Part print with two shaded views. Sizes in mm from the minimum x, y, z corner. Round coordinates to 2 decimals unless told otherwise and drop trailing zeros. Order: outer loops, then holes, each group sorted by start corner. A loop starts at its lowest first (then second) coordinate and runs counter-clockwise, first axis right, second up. Notation, with made-up numbers: M 61,5.5 L 110,5.5 A25 cw 110,29.5 Z; hole C -37,12 d6. An arc over 180 degrees is marked long. Answer as a JSON object with one key per item and string values.
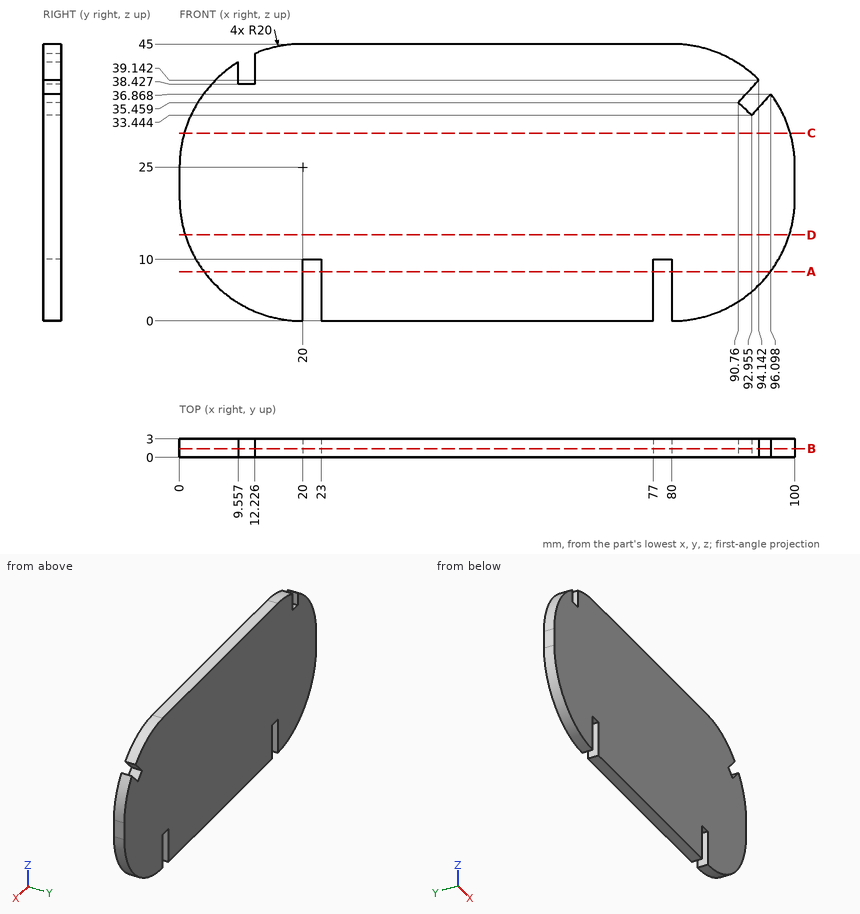
Item 1: Saw through at A-A on z = 8. List the corners of the cut face in (x, y).
Worked answers:
{"outline": "M 4,0 L 20,0 L 20,3 L 4,3 Z; M 23,0 L 77,0 L 77,3 L 23,3 Z; M 80,0 L 96,0 L 96,3 L 80,3 Z"}
Item 2: Drop flat-ended pins along their axis: pin 1 Ø1.5 at (y, z) = (1, 41) entering from -X; pin 2 Ø1.5 at (y, z) = (2, 7) entering from +X; pin 3 Ø1 at (y, z) = (1.5, 14) entering from -X. Give the stop position or say it passes through.
Worked answers:
{"pin 1": "stops at x = 7.06", "pin 2": "stops at x = 95.81", "pin 3": "stops at x = 0.77"}
Item 3: Saw through at B-B on y = 1.45. List the corners of the cut face in (x, z) (1 decimal).
Worked answers:
{"outline": "M 0,20 A20 ccw 20,0 L 20,10 L 23,10 L 23,0 L 77,0 L 77,10 L 80,10 L 80,0 A20 ccw 100,20 L 100,25 A20 ccw 96.1,36.9 L 93,33.4 L 90.8,35.5 L 94.1,39.1 A20 ccw 80,45 L 20,45 A20 ccw 12.2,43.4 L 12.2,38.4 L 9.6,38.4 L 9.6,42.1 A20 ccw 0,25 Z"}
Item 4: Saw through at D-D on z = 14. List the corners of the cut face in (x, y).
Worked answers:
{"outline": "M 0.92,0 L 99.08,0 L 99.08,3 L 0.92,3 Z"}
Item 5: Saw through at C-C on z = 30.5. List the corners of the cut face in (x, y).
Worked answers:
{"outline": "M 0.77,0 L 99.23,0 L 99.23,3 L 0.77,3 Z"}
Item 6: Wall check: line 1 along X through (y, z) = (0.5, 5); line 2 along X through (y, z) = (1.65, 3) (1 decimal); line 3 along X through (y, z) = (0.8, 25.5). Give the ranges that are in metal, low to high. Write a range as [from, to].
Worked answers:
{"line 1": "x = [6.77, 20], [23, 77], [80, 93.23]", "line 2": "x = [9.5, 20], [23, 77], [80, 90.5]", "line 3": "x = [0.01, 99.99]"}
